Autodesk Inventor part; units mm, degrees
ref_plane "YZ Plane" through (0, 0, 0) normal (1, 0, 0) x (0, 1, 0)
ref_plane "XZ Plane" through (0, 0, 0) normal (0, 1, 0) x (-1, 0, 0)
ref_plane "XY Plane" through (0, 0, 0) normal (0, 0, 1) x (1, 0, 0)
sketch "Sketch1" plane through (0, 0, 0) normal (0, 1, 0) x (-1, 0, 0)
  line L0 (0, 0) -> (-1016, 0)
  line L1 (-1016, 0) -> (-1016, -1930.4)
  line L2 (-1016, -1930.4) -> (0, -1930.4)
  line L3 (0, -1930.4) -> (0, 0)
  dimension "d0" = 1016
  dimension "d1" = 1930.4
extrude "Extrusion1" add sketch "Sketch1" against normal blind 152.4
sketch "Sketch2" plane through (0, -152.4, 0) normal (0, -1, 0) x (1, 0, 0)
  line L0 (25.4, -25.4) -> (990.6, -25.4)
  line L1 (990.6, -25.4) -> (990.6, -1905)
  line L2 (990.6, -1905) -> (25.4, -1905)
  line L3 (25.4, -1905) -> (25.4, -25.4)
  line L4 (25.4, -965.2) -> (0, -965.2)
  line L5 (0, 0) -> (0, -1930.4)
  line L6 (508, -1905) -> (508, -1930.4)
  line L7 (0, -1930.4) -> (1016, -1930.4)
  line L8 (990.6, -965.2) -> (1016, -965.2)
  line L9 (1016, -1930.4) -> (1016, 0)
  line L10 (508, -25.4) -> (508, 0)
  line L11 (1016, 0) -> (0, 0)
  dimension "d4" = 25.4
  dimension "d5" = 25.4
extrude "Extrusion2" cut sketch "Sketch2" against normal blind 50.8 contours L0 L1 L2 L3
sketch "Sketch3" plane through (0, -101.6, 0) normal (0, -1, 0) x (1, 0, 0)
  line L0 (990.6, -25.4) -> (990.6, -1905)
  line L1 (990.6, -279.4) -> (965.2, -279.4)
  line L2 (965.2, -279.4) -> (965.2, -736.6)
  line L3 (965.2, -736.6) -> (990.6, -736.6)
  line L4 (990.6, -736.6) -> (990.6, -279.4)
  line L5 (25.4, -1905) -> (25.4, -25.4)
  line L6 (990.6, -1905) -> (25.4, -1905)
  line L7 (990.6, -25.4) -> (990.6, -1905)
  line L8 (25.4, -25.4) -> (990.6, -25.4)
  line L9 (990.6, -1651) -> (965.2, -1651)
  line L10 (965.2, -1651) -> (965.2, -1193.8)
  line L11 (965.2, -1193.8) -> (990.6, -1193.8)
  line L12 (990.6, -1193.8) -> (990.6, -1651)
  point P0 (0, 0)
  dimension "d8" = 25.4
  dimension "d9" = 457.2
  dimension "d10" = 254
  dimension "d11" = 25.4
  dimension "d12" = 457.2
  dimension "d13" = 254
extrude "Extrusion3" cut sketch "Sketch3" against normal blind 50.8 contours L0 L3 L2 L1 | L0 L9 L10 L11
ref_plane "Work Plane1" through (508, 0, 0) normal (1, 0, 0) x (0, 0, -1)
mirror "Mirror1" about plane through (508, 0, 0) normal (1, 0, 0) of "Extrusion3"
sketch "Sketch4" plane through (0, -101.6, 0) normal (0, -1, 0) x (1, 0, 0)
  line L0 (25.4, -25.4) -> (990.6, -25.4)
  line L1 (812.8, -25.4) -> (660.4, -25.4)
  line L2 (660.4, -25.4) -> (660.4, -50.8)
  line L3 (660.4, -50.8) -> (812.8, -50.8)
  line L4 (812.8, -50.8) -> (812.8, -25.4)
  line L5 (355.6, -25.4) -> (203.2, -25.4)
  line L6 (203.2, -25.4) -> (203.2, -50.8)
  line L7 (203.2, -50.8) -> (355.6, -50.8)
  line L8 (355.6, -50.8) -> (355.6, -25.4)
  line L9 (990.6, -25.4) -> (990.6, -1905)
  line L10 (25.4, -1905) -> (25.4, -25.4)
  point P0 (0, 0)
  dimension "d16" = 152.4
  dimension "d17" = 25.4
  dimension "d18" = 152.4
  dimension "d19" = 25.4
  dimension "d20" = 177.8
  dimension "d21" = 177.8
extrude "Extrusion4" cut sketch "Sketch4" against normal blind 50.8
ref_plane "Work Plane2" through (0, 0, -965.2) normal (0, 0, 1) x (1, 0, 0)
mirror "Mirror2" about plane through (0, 0, -965.2) normal (0, 0, 1) of "Extrusion4"
properties part number "rev1 top"
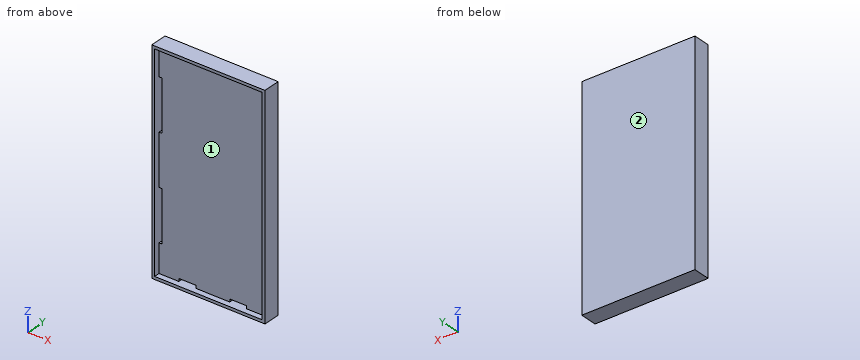
Read the model definition and answer for the solid it produces. Units are mm, in the model's axes. Face numbers are marked on the shaded views. Give positions to 0.01 mm unless a question says otherwise; leave off trailing zeros. Write each loop counter-clockwise with the first axis right and the second up, starting at its lowest first coordinate (ties: lowest second). Pieces come first, ordered by that corner, then holes. Notation, with made-up numbers: (32.5, -27) -> (84.5, -27) arc R19 cw to (84.5, -4) -> close; hole circle Ø8 at (-5, 75). An arc over 180 degrees is marked (long way). Answer as a JSON object with one key per item and string values. Group by question number.
1) Each of these flat-tipped pins is pushed along its axis until it touches: P1, Ø20.5, axis at y = -84, z = -1896, coming from the -X side; P2, Ø12, axis at x = 333, z = -1257, coming from the -Y side; P3, Ø7.5, axis at x = 746.5, z = -1890, coming from the -Y side. Where does it stop, or does it pass through?
2) Find section A-A (y = -129.5). Write down the section's boundary in (x, z).
3) Find section D-D (x = 395). Write down the section's boundary in (y, z), and give its area (3 significant figures).
4) Find section C-C (z = -1406.5). Write down the section's boundary in (x, y), and give its area (3 significant figures).
5) Consider L1, parallel to Z at x = 665, y = -56; L2, parallel to X at y = -67, z = -1531.5; L3, parallel to Z at x = 153, y = -102. Determine where each line is inside the solid, lowest interval first. Write a range as from..to.
6) The mould has two halves that part along X. Classify the marked faces 1 and 2: +X half, -X half, draft (parallel to the pull), parting line (faces both ways), or undercut.
7) Find section B-B (x = 239). Write down the section's boundary in (y, z).
Values follow:
{
 "1": {"P1": "stops at x = 0", "P2": "stops at y = -101.6", "P3": "stops at y = -50.8"},
 "2": {"outline": "(0, -1930.4) -> (1016, -1930.4) -> (1016, 0) -> (0, 0) -> close; hole (25.4, -1905) -> (990.6, -1905) -> (990.6, -25.4) -> (25.4, -25.4) -> close"},
 "3": {"outline": "(-152.4, -1930.4) -> (0, -1930.4) -> (0, 0) -> (-152.4, 0) -> (-152.4, -25.4) -> (-101.6, -25.4) -> (-101.6, -1905) -> (-152.4, -1905) -> close", "area": "199,000 mm2"},
 "4": {"outline": "(0, -152.4) -> (25.4, -152.4) -> (25.4, -50.8) -> (50.8, -50.8) -> (50.8, -101.6) -> (965.2, -101.6) -> (965.2, -50.8) -> (990.6, -50.8) -> (990.6, -152.4) -> (1016, -152.4) -> (1016, 0) -> (0, 0) -> close", "area": "103,000 mm2"},
 "5": {"L1": "z = -1930.4..-1905, -1879.6..-50.8, -25.4..0", "L2": "x = 0..25.4, 50.8..965.2, 990.6..1016", "L3": "z = -1930.4..-1905, -25.4..0"},
 "6": {"face 1": "undercut", "face 2": "draft"},
 "7": {"outline": "(-152.4, -1930.4) -> (0, -1930.4) -> (0, 0) -> (-152.4, 0) -> (-152.4, -25.4) -> (-50.8, -25.4) -> (-50.8, -50.8) -> (-101.6, -50.8) -> (-101.6, -1879.6) -> (-50.8, -1879.6) -> (-50.8, -1905) -> (-152.4, -1905) -> close"}
}
